Can you work these out from the model? Positions are in its coordinate system, mm. A direction names the side the tool comes from. Give positions to 0.01 mm unless a question says otherwise; leave off trailing zeros. Order: outer loops, then holes, each group sorted by start corner. A loop starts at its lowest first (then second) coordinate and runs counter-clockwise, first axis right, second up. Notation, with made-up numbers: M 51.25,-36 L 110.25,-36 A25 ccw 110.25,-20 Z; hole C 82.25,83 d8. An arc over 180 degrees is marked long. One line per question, with ' | ' between items. Start each with the question number.
1) If we section it at A-A, the plane x = 7: Please give me the cut outline in (y, z) (3 decimals), plus the area to 3 significant figures.
2) I'm going to push flat-ended pins straight in: pin 1 Ø8 at (x, y) = (-8, -5) entering from +Z; pin 2 Ø8 at (x, z) = (-0.5, 42) entering from +Y; pin 3 Ø4 at (x, z) = (0, 82.55) entering from -Y. Where does each tip first touch, or does it pass through?
3) If we section it at D-D, the plane z = 82.55: Please give me the cut outline in (x, y) (3 decimals), plus the area to 3 significant figures.
4) Please list where these lines run through material, in increasing order: line 1 along Y through (x, z) = (-6.75, -14) (3 decimals); line 2 along Z through (x, y) = (0, 11.6) (3 decimals). Write a range as [from, to].
5) If we section it at B-B, the plane z = -88.9: Please give me the cut outline in (x, y) (3 decimals), plus the area to 3 significant figures.
6) For faces 1 (the flat face through (0, -9.525, -1)), 2 (the flat face through (0, 38.1, -89)), which set-ups out of +Z, -Z, +X, -X, +Y, -Y let a thin tool reach every point of the face, with its end or its side?
7) Thinking about a two-plate mould opening in Z: for faces 3 (the cylindrical face through (1.707, 25.222, -86.223)), 4 (the cylindrical face through (1.707, 11.135, 79.873)), 5 (the flat face through (11, 0, 101.6)), which applies, +Z half, -Z half, draft (parallel to the pull), parting line (faces both ways), or undercut?
Autodesk Inventor part; units mm, degrees
ref_plane "YZ Plane" through (0, 0, 0) normal (1, 0, 0) x (0, 1, 0)
ref_plane "XZ Plane" through (0, 0, 0) normal (0, 1, 0) x (-1, 0, 0)
ref_plane "XY Plane" through (0, 0, 0) normal (0, 0, 1) x (1, 0, 0)
sketch "Sketch1" plane through (0, 0, 0) normal (0, 0, 1) x (1, 0, 0)
  line L0 (-12.7, -12.7) -> (12.7, -12.7)
  line L1 (12.7, -12.7) -> (12.7, 12.7)
  line L2 (12.7, 12.7) -> (-12.7, 12.7)
  line L3 (-12.7, 12.7) -> (-12.7, -12.7)
  line L4 (-12.7, -12.7) -> (12.7, 12.7) construction
  line L5 (12.7, -12.7) -> (-12.7, 12.7) construction
  line L6 (-9.525, -9.525) -> (9.525, -9.525)
  line L7 (9.525, -9.525) -> (9.525, 9.525)
  line L8 (9.525, 9.525) -> (-9.525, 9.525)
  line L9 (-9.525, 9.525) -> (-9.525, -9.525)
  line L10 (-9.525, -9.525) -> (9.525, 9.525) construction
  line L11 (9.525, -9.525) -> (-9.525, 9.525) construction
  point P0 (0, 0)
  dimension "d0" = 3.175
  dimension "d1" = 25.4
extrude "Extrusion1" add sketch "Sketch1" along normal mid plane 203.2
sketch "Sketch2" plane through (-12.7, 12.7, 101.6) normal (0, 1, 0) x (1, 0, 0)
  line L0 (0, 203.2) -> (25.4, 203.2) construction
  line L1 (12.7, 203.2) -> (12.7, 0) construction
  line L2 (22.225, 0) -> (3.175, 0) construction
  circle A0 centre (12.7, 19.05) radius 3.175
  line L3 (25.4, 0) -> (0, 0)
  point P0 (12.7, 101.6)
  dimension "d4" = 6.35
  dimension "d5" = 19.05
extrude "Extrusion2" cut sketch "Sketch2" against normal through all
sketch "Sketch3" plane through (-12.7, 12.7, 101.6) normal (0, 1, 0) x (1, 0, 0)
  line L0 (0, 203.2) -> (25.4, 203.2) construction
  line L1 (12.7, 203.2) -> (12.7, 0) construction
  line L2 (25.4, 0) -> (0, 0) construction
  circle A0 centre (12.7, 190.5) radius 3.175
  point P0 (12.7, 101.6)
  dimension "d8" = 6.35
  dimension "d9" = 12.7
extrude "Extrusion3" add sketch "Sketch3" along normal blind 25.4
properties part number "1x1x8 Rectangular Tubing"
Results found:
1) outline: M -12.7,-101.6 L -9.525,-101.6 L -9.525,101.6 L -12.7,101.6 Z; M 9.525,-101.6 L 12.7,-101.6 L 12.7,101.6 L 9.525,101.6 Z | area: 1,290 mm²
2) pin 1: stops at z = 101.6 | pin 2: stops at y = 12.7 | pin 3: passes through
3) outline: M -12.7,-12.7 L -3.175,-12.7 L -3.175,-9.525 L -9.525,-9.525 L -9.525,9.525 L -3.175,9.525 L -3.175,12.7 L -12.7,12.7 Z; M 3.175,-12.7 L 12.7,-12.7 L 12.7,12.7 L 3.175,12.7 L 3.175,9.525 L 9.525,9.525 L 9.525,-9.525 L 3.175,-9.525 Z | area: 242 mm²
4) line 1: y = [-12.7, -9.525], [9.525, 12.7] | line 2: z = [-101.6, 79.375], [85.725, 101.6]
5) outline: M -12.7,-12.7 L 12.7,-12.7 L 12.7,12.7 L 3.175,12.7 L 3.175,38.1 L -3.175,38.1 L -3.175,12.7 L -12.7,12.7 Z; hole M -9.525,-9.525 L 9.525,-9.525 L 9.525,9.525 L -9.525,9.525 Z | area: 444 mm²
6) face 1: +Z, -Z | face 2: +Z, -Z, +X, -X, +Y
7) face 3: parting line | face 4: undercut | face 5: +Z half
